```python
from build123d import *

# Parameters (mm, degrees)
BOSS_EXTRUDE1_DEPTH = 28.575
FILLET1_R           = 2.54
FILLET2_R           = 2.54
SKETCH2_R           = 2.4892
CUT_EXTRUDE1_DEPTH  = 4.175


with BuildPart() as part:
    # Sketch1 → Boss-Extrude1 (new body, symmetric)
    with BuildSketch(Plane.XY):
        Polygon((76.2, 0), (73.599192259, 1.821105185), (74.547199614, 3.175), (0, 3.175), (0, 0), align=None)
        Polygon((76.2, 3.175), (76.2, 0), (105.337682967, 41.61292385), (102.736875226, 43.434029035), (74.547199614, 3.175), align=None)
        Polygon((74.547199614, 3.175), (73.599192259, 1.821105185), (76.2, 0), (76.2, 3.175), align=None)
    extrude(amount=BOSS_EXTRUDE1_DEPTH, both=True)

    # Fillet1
    fillet1_edges = [part.edges().sort_by_distance(p)[0] for p in [
        (74.547199614, 3.175, 0),
    ]]
    fillet(fillet1_edges, radius=FILLET1_R)

    # Fillet2
    fillet2_edges = [part.edges().sort_by_distance(p)[0] for p in [
        (76.2, 0, 0),
    ]]
    fillet(fillet2_edges, radius=FILLET2_R)

    # Sketch2 → Cut-Extrude1 (cut, through all)
    with BuildSketch(Plane(origin=(0, 3.175, 0), x_dir=(1, 0, 0), z_dir=(0, 1, 0))):
        with Locations((60.524959306, -15.875)):
            Circle(SKETCH2_R)
        with Locations((22.424959306, -15.875)):
            Circle(SKETCH2_R)
    extrude(amount=-CUT_EXTRUDE1_DEPTH, mode=Mode.SUBTRACT)


solid = part.part
```
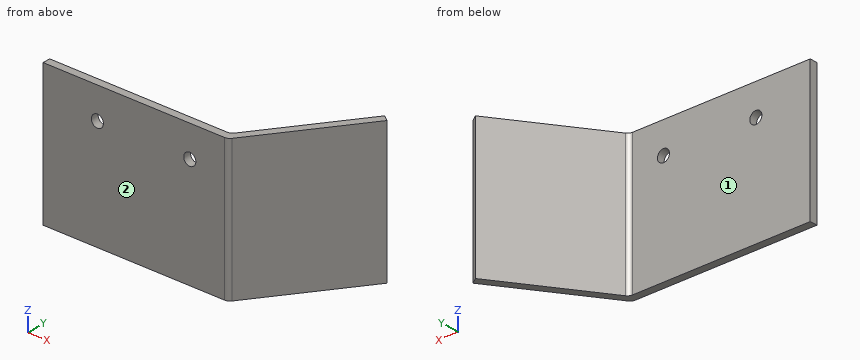
Part model, mm, in its own coordinate system. Face numbers are marked on the shaded views. A direction names the side the tool comes from. Give positions to 0.01 mm unless a question says otherwise; leave off trailing zeros. Order: outer loops, then holes, each group sorted by start corner. A loop starts at its lowest first (then second) coordinate and runs counter-clockwise, first axis right, second up. Notation, with made-up numbers: M 78.25,-33 L 137.25,-33 A31 ccw 137.25,-1 Z; hole C 45.25,21 d4. An arc over 180 degrees is marked long. Use a Markdown table: item, result. Add a question column.
(1) Saw through at C-C, the plane y = 21.5. Give the cut face in (x, z) (1 decimal).
(2) Probe line 1 along Y through (x, z) = (27.5, -21) (3 decimals); line 2 along X through (y, z) = (7, -19.5); line 3 along X through (y, z) = (11, 22.5). List the from-to ranges inside material, lowest first. Write a range as [from, to].
(3) Saw through at A-A, the plane z = 24.5. Give the cut face in (x, y) (3 decimals).
(4) 3-axis set-ups, long thin cutter, end or side, ignore diameter. For the marked faces 1 and 2: which of +Z, -Z, +X, -X, +Y, -Y reach the whole face in a straight line?
(5) Drop flat-ended pins along their axis: P1, Ø1.5, axis at y = 33, z = -8, coming from the +X side; P2, Ø8, axis at x = 60.52, z = 15.88, coming from the +Y side (3 decimals); P3, Ø10, axis at y = 16.5, z = 14.5, coming from the -X side. Give the stop position or say it passes through.
(6) Saw through at B-B, the plane x = 31. Give the cut face in (y, z) (3 decimals).
Answer key:
| question | item | result |
|---|---|---|
| 1 | outline | M 87.4,-28.6 L 91.3,-28.6 L 91.3,28.6 L 87.4,28.6 Z |
| 2 | line 1 | [0, 3.175] |
| 2 | line 2 | [77.23, 81.1] |
| 2 | line 3 | [80.03, 83.9] |
| 3 | outline | M 0,0 L 74.878,0 A2.54 ccw 76.958,1.083 L 105.338,41.613 L 102.737,43.434 L 75.306,4.258 A2.54 cw 73.225,3.175 L 0,3.175 Z |
| 4 | face 1 | +Z, -Z, -X, +Y |
| 4 | face 2 | +Z, -Z, +X, -X, -Y |
| 5 | P1 | x = 99.83 |
| 5 | P2 | y = 3.175 |
| 5 | P3 | x = 80.38 |
| 6 | outline | M 0,-28.575 L 3.175,-28.575 L 3.175,28.575 L 0,28.575 Z |
